Source: CAD feature listing. Evaluate the final solid. Frame: model axes, mm. Give positions to 0.01 mm unless a question says otherwise; leave off trailing zeros. Write each loop counter-clockwise with the first axis right and the second up, starting at its lowest first coordinate (ties: lowest second). Pieces come first, ordered by that corner, then holes. Notation, with made-up numbers: (8.5, 18.25) - (55.5, 18.25) arc R17 ccw to (55.5, 45.25) - close; hole circle Ø7 at (20.25, 62.5). An arc over 180 degrees is marked (long way). Answer as a JSON object with one key per item and string values. Group by question number.
from build123d import *

# Parameters (mm, degrees)
BOSS_EXTRUDE1_DEPTH = 1000


with BuildPart() as part:
    # Sketch1 → Boss-Extrude1 (new body)
    with BuildSketch(Plane.XY):
        with BuildLine():
            Line((-119.957004607, 72.181122853), (82.042995393, 72.181122853))
            ThreePointArc((82.042995393, 72.181122853), (109.042995393, 45.181122853), (82.042995393, 18.181122853))
            Line((82.042995393, 18.181122853), (-119.957004607, 18.181122853))
            Line((-119.957004607, 18.181122853), (-119.957004607, 44.181122853))
            Line((-119.957004607, 44.181122853), (-117.957004607, 44.181122853))
            Line((-117.957004607, 44.181122853), (-117.957004607, 20.181122853))
            Line((-117.957004607, 20.181122853), (82.042995393, 20.181122853))
            ThreePointArc((82.042995393, 20.181122853), (107.042995393, 45.181122853), (82.042995393, 70.181122853))
            Line((82.042995393, 70.181122853), (-117.957004607, 70.181122853))
            Line((-117.957004607, 70.181122853), (-117.957004607, 46.181122853))
            Line((-117.957004607, 46.181122853), (-119.957004607, 46.181122853))
            Line((-119.957004607, 46.181122853), (-119.957004607, 72.181122853))
        make_face()
    extrude(amount=-BOSS_EXTRUDE1_DEPTH)


solid = part.part
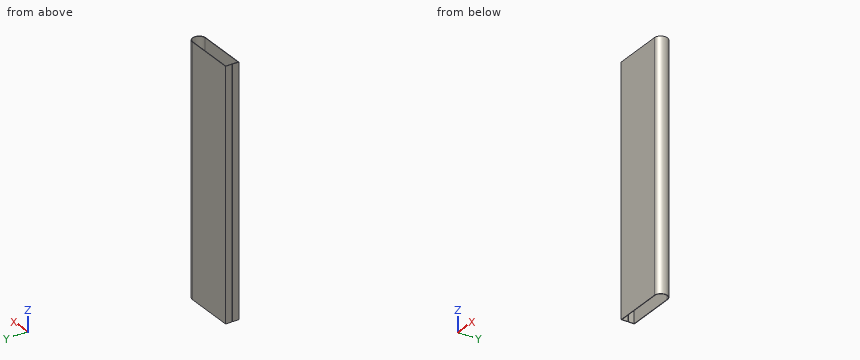
Q1. First-contact query: pin 1 Ø19 at (y, z) = (28.5, -746.5) entering from +X; pin 2 Ø8 at (x, y) = (-58.5, 65) entering from -Z; pin 3 Ø6 at (y, z) = (31.5, -268.5) entering from +X; pin 4 Ø19 at (y, z) = (63.5, -353) entering from +X. Flat tips, straight axial feed; report the tip coordinate or a pass-through.
Q2. Section C-C on y = 58.5. Return the cut outline in (x, z), then the cut area to 3 significant figures.
Q3. Section A-A on x = 44. Return the cut outline in (y, z), then the cut area to 3 significant figures.
Q4. Ray query, probe 1 along Y at (x, z) = (47, -489.5); probe 2 along X at (y, z) = (46, -695.5); probe 3 along X at (y, z) = (42, -651.5). Return the intervals inside material, ascending. Write a range as [from, to].
Q5. Section B-B on z = -923. Return the cut outline in (x, y).
Taken from the geometry:
{
 "1": {"pin 1": "stops at x = 108.07", "pin 2": "passes through", "pin 3": "stops at x = 106.84", "pin 4": "stops at x = 107.56"},
 "2": {"outline": "(-119.96, -1000) - (-117.96, -1000) - (-117.96, 0) - (-119.96, 0) - close; (103.2, -1000) - (105.53, -1000) - (105.53, 0) - (103.2, 0) - close", "area": "4,330 mm²"},
 "3": {"outline": "(18.18, -1000) - (20.18, -1000) - (20.18, 0) - (18.18, 0) - close; (70.18, -1000) - (72.18, -1000) - (72.18, 0) - (70.18, 0) - close", "area": "4,000 mm²"},
 "4": {"probe 1": "y = [18.18, 20.18], [70.18, 72.18]", "probe 2": "x = [107.03, 109.03]", "probe 3": "x = [-119.96, -117.96], [106.84, 108.85]"},
 "5": {"outline": "(-119.96, 18.18) - (82.04, 18.18) arc R27 ccw to (82.04, 72.18) - (-119.96, 72.18) - (-119.96, 46.18) - (-117.96, 46.18) - (-117.96, 70.18) - (82.04, 70.18) arc R25 cw to (82.04, 20.18) - (-117.96, 20.18) - (-117.96, 44.18) - (-119.96, 44.18) - close"}
}
